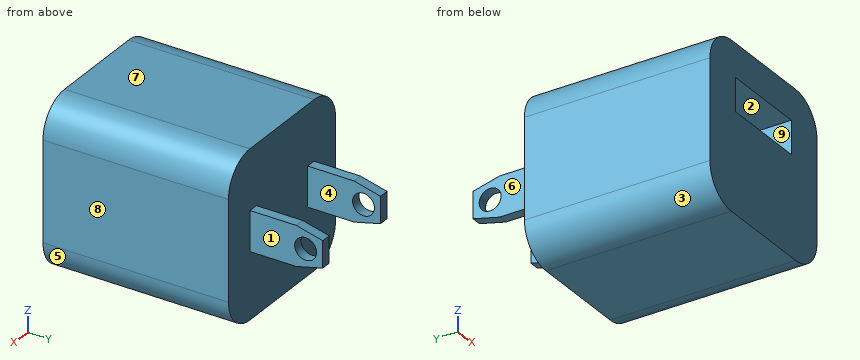
```python
from build123d import *

# Parameters (mm, degrees)
F0_W      = 25
F0_H      = 25
F1_DEPTH  = 14
F3_DEPTH  = 15
F4_W      = 1.5
F4_H      = 6
F5_DEPTH  = 11
F6_R      = 1.65
F7_DEPTH  = 30.4
F8_R      = 5
F9_W      = 8.8653210551
F9_H      = 1.5135915019
F10_DEPTH = 10


with BuildPart() as f1:
    # F0 (on Front) → F1 (new body, symmetric)
    with BuildSketch(Plane.XZ):
        Rectangle(F0_W, F0_H)
    extrude(amount=F1_DEPTH, both=True)

    # F2 (on face) → F3 (cut)
    with BuildSketch(Plane.XZ.offset(14)):
        Polygon((-6.5, 2.5), (0, 2.5), (6.5, 2.5), (6.5, 7.5), (-6.5, 7.5), align=None)
    extrude(amount=-F3_DEPTH, mode=Mode.SUBTRACT)

    # F4 (on face) → F5 (join)
    with BuildSketch(Plane(origin=(0, 14, 0), x_dir=(-1, 0, 0), z_dir=(0, 1, 0))):
        with Locations((-6.75, 0.5)):
            Rectangle(F4_W, F4_H)
        with Locations((6.75, 0.5)):
            Rectangle(F4_W, F4_H)
    extrude(amount=F5_DEPTH)

    # F6 (on face) → F7 (cut)
    with BuildSketch(Plane.YZ.offset(7.5)):
        with Locations((22.4171727896, 0.5)):
            Circle(F6_R)
        Polygon((25, 2.4996667635), (25, 3.5), (21, 3.5), align=None)
        Polygon((25, -2.5), (25, -1.5), (21, -2.5), align=None)
    extrude(amount=-F7_DEPTH, mode=Mode.SUBTRACT)

    # F8
    f8_edges = [f1.edges().sort_by_distance(p)[0] for p in [
        (-12.5, 0, 12.5),
        (12.5, 0, 12.5),
        (12.5, 0, -12.5),
        (-12.5, 0, -12.5),
    ]]
    fillet(f8_edges, radius=F8_R)

    # F9 (on face) → F10 (join)
    with BuildSketch(Plane.XZ.offset(-1)):
        with Locations((0.1513590105, 5.6867792737)):
            Rectangle(F9_W, F9_H)
    extrude(amount=F10_DEPTH)


solid = f1.part
```
CAD build for the part. Positions are in the model's coordinates, mm. Face numbers are marked on the shaded views. A direction names the side the tool comes from. Give positions to 0.01 mm unless a question says otherwise; leave off trailing zeros. Order: outer loops, then holes, each group sorted by start corner. A loop starts at its lowest first (then second) coordinate and runs counter-clockwise, first axis right, second up. Notation, with made-up numbers: M -39,16.25 L -14,16.25 A26 ccw -14,34.25 Z; hole C -5.5,-33.5 d5. An arc over 180 degrees is marked long. Put each result on its own line as item: value. Start each with the question number.
(1) Mould opens along X. For the marked faces 6, 7, 8 and 9 say: +X half, -X half, draft (parallel to the pull), parting line (faces both ways), or undercut.
(2) Saw through at D-D, the plane x = -3.5. Write the cut outline in (y, z), then the cut area to 3 significant figures.
(3) Saw through at B-B, the plane z = 0.5. Write the cut outline in (x, y).
(4) Flat gauge pins, fed straight in: pin 1 Ø1.2 at (x, y) = (7, 19) entering from +Z; pin 2 Ø0.8 at (x, y) = (-7, 18.5) entering from -Z; pin 3 Ø5 at (y, z) = (17.5, 0) entering from +X; pin 4 Ø3 at (y, z) = (22.42, 0.5) entering from +X. Where does each tip first touch, or does it go through?
(5) Drill centre lines: line 1 along Z through (x, y) = (1.25, -1); line 2 along X through (y, z) = (20, 2.75); line 3 along Z through (x, y) = (-5.5, -9.5). Where is each one in solid material? Low to high.
(6) Which spindle directions (+Z, -Z, +X, -X, +Y, -Y) get a long thin tool onto all of the face, cutting with end or side? Do the marked faces 1, 2, 3, 4 and 5. Say none if no direction does.
(7) Saw through at A-A, the plane y = 14.5. Write the cut outline in (x, z).
(8) Saw through at C-C, the plane y = 3. Write the cut outline in (x, z), then the cut area to 3 significant figures.
Check result:
1. face 6: -X half
1. face 7: draft
1. face 8: +X half
1. face 9: undercut
2. outline: M -14,-12.5 L 14,-12.5 L 14,12.5 L -14,12.5 L -14,7.5 L 1,7.5 L 1,6.44 L -9,6.44 L -9,4.93 L 1,4.93 L 1,2.5 L -14,2.5 Z
2. area: 640 mm2
3. outline: M -12.5,-14 L 12.5,-14 L 12.5,14 L 7.5,14 L 7.5,20.77 L 6,20.77 L 6,14 L -6,14 L -6,20.77 L -7.5,20.77 L -7.5,14 L -12.5,14 Z; M -7.5,24.07 L -6,24.07 L -6,25 L -7.5,25 Z; M 6,24.07 L 7.5,24.07 L 7.5,25 L 6,25 Z
4. pin 1: stops at z = 3.5
4. pin 2: stops at z = -2.5
4. pin 3: stops at x = 7.5
4. pin 4: passes through
5. line 1: z = -12.5 to 2.5, 4.93 to 6.44, 7.5 to 12.5
5. line 2: x = -7.5 to -6, 6 to 7.5
5. line 3: z = -12.5 to 2.5, 7.5 to 12.5
6. face 1: +Z, -Z, +X, +Y
6. face 2: -Y
6. face 3: -Z, -X, +Y, -Y
6. face 4: +Z, -Z, +Y
6. face 5: -Z, +X, +Y, -Y
7. outline: M -7.5,-2.5 L -6,-2.5 L -6,3.5 L -7.5,3.5 Z; M 6,-2.5 L 7.5,-2.5 L 7.5,3.5 L 6,3.5 Z
8. outline: M -12.5,-7.5 A5 ccw -7.5,-12.5 L 7.5,-12.5 A5 ccw 12.5,-7.5 L 12.5,7.5 A5 ccw 7.5,12.5 L -7.5,12.5 A5 ccw -12.5,7.5 Z
8. area: 604 mm2
